```python
from build123d import *

# Parameters (mm, degrees)
SKETCH152_W             = 30
SKETCH152_H             = 45
PAD076_DEPTH            = 4
PAD077_DEPTH            = 20
SKETCH159_R             = 1.6
POCKET059_DEPTH         = 5
FILLET_R                = 6
CHAMFER_SIZE            = 2
FILLET001_R             = 5
SKETCH_R                = 1.35
POCKET_DEPTH            = 19.001
POCKET_DEPTH_BACK       = -11.001
SKETCH165_R             = 2.95
POCKET060_DEPTH         = 5
SKETCH166_R             = 1.55
POCKET061_DEPTH         = 2.5
BODY061_ROLL_ANGLE      = -90
BODY061_PLACEMENT_ANGLE = -90


with BuildPart() as part:
    # Sketch152 → Pad076 (new body)
    with BuildSketch(Plane.XY):
        with Locations((15, 22.5)):
            Rectangle(SKETCH152_W, SKETCH152_H)
    extrude(amount=PAD076_DEPTH)

    # Sketch153 (on Face1 of Pad076) → Pad077 (join)
    with BuildSketch(Plane.XZ):
        with BuildLine():
            ThreePointArc((30, 22.999996), (26.937338, 32.08295), (19, 37.456832))
            Line((19, 37.456832), (19, 41.456832))
            Line((19, 41.456832), (16.5, 41.456832))
            Line((16.5, 35.30894), (16.5, 41.456832))
            ThreePointArc((13.5, 35.30894), (15, 10.6), (16.5, 35.30894))
            Line((13.5, 41.456832), (13.5, 35.30894))
            Line((13.5, 41.456832), (11, 41.456832))
            Line((11, 41.456832), (11, 37.456832))
            ThreePointArc((11, 37.456832), (3.062664, 32.082951), (0, 23))
            Line((0, 0), (0, 23))
            Line((0, 0), (30, 0))
            Line((30, 22.999996), (30, 0))
        make_face()
    extrude(amount=PAD077_DEPTH)

    # Sketch159 → Pocket059 (cut)
    with BuildSketch(Plane.XY.offset(4)):
        with Locations((7.5, 36.5)):
            Circle(SKETCH159_R)
        with Locations((15, 23.5)):
            Circle(SKETCH159_R)
        with Locations((22.5, 36.5)):
            Circle(SKETCH159_R)
        with Locations((26.5, 30)):
            Circle(SKETCH159_R)
    extrude(amount=-POCKET059_DEPTH, mode=Mode.SUBTRACT)

    # Sketch164 (on DatumPlane) → Groove (revolve, cut)
    with BuildSketch(Plane(origin=(15, 0, 0), x_dir=(0, -1, 0), z_dir=(-1, 0, 0))):
        with BuildLine():
            Line((42.60314, 23.220009), (24.100682, 23.220009))
            ThreePointArc((24.100682, 23.220009), (15.81151, 41.734328), (-2.093555, 51.268426))
            Line((-2.093555, 59.264427), (-2.093555, 51.268426))
            Line((-2.093555, 59.264427), (35.073817, 59.264427))
            Line((42.60314, 23.220009), (35.073817, 59.264427))
        make_face()
    revolve(axis=Axis((15, 0, 22.999996), (0, -1, 0)), mode=Mode.SUBTRACT)

    # Fillet
    fillet_edges = [part.edges().sort_by_distance(p)[0] for p in [
        (15, 0, 4),
    ]]
    fillet(fillet_edges, radius=FILLET_R)

    # Chamfer
    chamfer_edges = [part.edges().sort_by_distance(p)[0] for p in [
        (12.25, 0, 41.456832),
        (17.75, 0, 41.456832),
    ]]
    chamfer(chamfer_edges, length=CHAMFER_SIZE)

    # Fillet001
    fillet001_edges = [part.edges().sort_by_distance(p)[0] for p in [
        (11, -9.399365, 37.456832),
        (19, -9.399365, 37.456832),
    ]]
    fillet(fillet001_edges, radius=FILLET001_R)

    # Sketch (on Face23 of Fillet001) → Pocket (cut, two sides)
    with BuildSketch(Plane.YZ.offset(19)) as pocket_sk:
        with Locations((-10, 38)):
            Circle(SKETCH_R)
    extrude(amount=-POCKET_DEPTH, mode=Mode.SUBTRACT)
    extrude(pocket_sk.sketch, amount=-POCKET_DEPTH_BACK, mode=Mode.SUBTRACT)

    # Sketch165 (on Face25 of Pocket) → Pocket060 (cut)
    with BuildSketch(Plane.YZ.offset(19)):
        with Locations((-10, 38)):
            Circle(SKETCH165_R)
    extrude(amount=POCKET060_DEPTH, mode=Mode.SUBTRACT)

    # Sketch166 (on Face31 of Pocket060) → Pocket061 (cut)
    with BuildSketch(Plane.YZ.offset(19)):
        with Locations((-10, 38)):
            Circle(SKETCH166_R)
    extrude(amount=-POCKET061_DEPTH, mode=Mode.SUBTRACT)


with BuildPart() as part_1:
    # Body061 roll: moved
    add(part.part.rotate(Axis((0, 0, 0), (1, 0, 0)), BODY061_ROLL_ANGLE))


with BuildPart() as part_2:
    # Body061 placement: moved
    add(part_1.part.rotate(Axis((0, 0, 0), (0, 0, 1)), BODY061_PLACEMENT_ANGLE))


solid = part_2.part
```
Model file for the job. Use its own axes, mm. A direction names the side the tool comes from. Coordinates: 2 decimals unless noted, no trailing zeros. Write each loop counter-clockwise with the first axis right and the second up, starting at its lowest first coordinate (ties: lowest second). Pieces come first, ordered by that corner, then holes. Notation, with made-up numbers: (-35.75, 53.25) - (-9.75, 53.25) arc R14 ccw to (-9.75, 80.25) - close; hole circle Ø11 at (-11.5, 43.5). An arc over 180 degrees is marked (long way). Use a Markdown table: item, result. Add a question column.
Item 1: Two-plate mould, pull along Z, no slides. Class faces 1 (the face through (2.03, -23.24, -35.08)), 2 (the face through (11.7, -9.4, 0)), 3 (the face through (38, -16.5, 8)): pulls with the +Z half, pulls with the -Z half, needs draft (parallel to the pull), parting line crosses it, or undercut.
Item 2: 3-axis set-ups, long thin cutter, end or side, ignore diameter. For faces 4 (the face through (4, -15, -26)), 5 (the face through (41.457, -12, 9)), 6 (the face through (35.052, -20.884, 10.12)), 7 (the face through (40, -13.5, 10)): which of +Z, -Z, +X, -X, +Y, -Y reach the whole face in a straight line?
Item 3: Band-saw the part on B-B, the plane z = -39.5. Write the cut outline in (x, y).
Item 4: Band-saw the part on A-A, the plane z = -23.5. Write the cut outline in (x, y), and give its area (3 significant figures).
Item 5: Band-saw the part on C-C, the plane y = -7.5. Give the number of separate pieces and of enclosed holes in the cut face, and give its area (3 significant figures).
Item 6: Drill centre lines: line 1 along Y through (x, z) = (1.15, -36.5); line 2 along X through (y, z) = (-12, -26.5); line 3 along Y through (x, z) = (26, 2.5). Where is each one in solid material? Low to high.
Item 7: Drop flat-ended pins along their axis: pin 1 (1.9 mm diameter, centred on y = -22.5, z = -36.5, fed in from +X) (1 decimal); pin 2 (2 mm diameter, centred on x = 29, z = 9.5, fed in from -Y); pin 3 (1.8 mm diameter, centred on x = 38.5, z = 12.5, fed in from -Y); pin 4 (7 mm diameter, centred on x = 37, z = 7.5, fed in from -Y). Give the stop position or say it passes through.
A:
| question | item | result |
|---|---|---|
| 1 | face 1 | undercut |
| 1 | face 2 | pulls with the -Z half |
| 1 | face 3 | needs draft |
| 2 | face 4 | -Z, +X, +Y, -Y |
| 2 | face 5 | +Z, -Z, +X, +Y, -Y |
| 2 | face 6 | -Y |
| 2 | face 7 | +Z, -Z, +X |
| 3 | outline | (0, -30) - (4, -30) - (4, 0) - (0, 0) - close |
| 4 | outline | (0, -30) - (4, -30) - (4, -16.6) - (0, -16.6) - close; (0, -13.4) - (4, -13.4) - (4, 0) - (0, 0) - close |
| 4 | area | 107 mm² |
| 5 | separate pieces | 3 |
| 5 | enclosed holes | 0 |
| 5 | area | 444 mm² |
| 6 | line 1 | y = -30 to -24.1, -20.9 to -9.1, -5.9 to 0 |
| 6 | line 2 | x = 0 to 4 |
| 6 | line 3 | y = -29.7 to -27.03, -2.97 to -0.3 |
| 7 | pin 1 | passes through |
| 7 | pin 2 | stops at y = -29.14 |
| 7 | pin 3 | stops at y = -20.12 |
| 7 | pin 4 | stops at y = -25.71 |
